```python
from build123d import *

# Parameters (mm, degrees)
BASPROSKE_W         = 15
BASPROSKE_H         = 20
TOOTHCUT_DEPTH      = 33.015621187
TEETHCUTS_COUNT     = 14
TEETHCUTS_ANGLE     = 334.285714286
BORSKE_R            = 2
BORE_DEPTH          = 50.0000508
SKETCH1_R           = 12.170076636
BOSS_EXTRUDE1_DEPTH = 20
SKETCH3_R           = 2
CUT_EXTRUDE1_DEPTH  = 45.828194428


with BuildPart() as part:
    # BasProSke → Base-Revolve (revolve)
    with BuildSketch(Plane(origin=(0, 0, 0), x_dir=(1, 0, 0), z_dir=(0, 1, 0)), mode=Mode.PRIVATE) as base_revolve_sk:
        with Locations((7.5, 10)):
            Rectangle(BASPROSKE_W, BASPROSKE_H)
    revolve(base_revolve_sk.sketch.rotate(Axis((-10, 0, 0), (1, 0, 0)), 180), axis=Axis((-10, 0, 0), (1, 0, 0)))

    # TooCutSke → ToothCut (cut, through all)
    with BuildSketch(Plane(origin=(0, 0, 0), x_dir=(0, 0, -1), z_dir=(1, 0, 0))):
        with BuildLine():
            ThreePointArc((1.339503949, 14.311450142), (0, 14.374), (-1.339503949, 14.311450142))
            ThreePointArc((-1.339503949, 14.311450142), (-2.055976555, 17.261705303), (-3.954182827, 19.631125371))
            ThreePointArc((-3.954182827, 19.631125371), (0, 20.0254), (3.954182827, 19.631125371))
            ThreePointArc((3.954182827, 19.631125371), (2.055976555, 17.261705303), (1.339503949, 14.311450142))
        make_face()
    toothcut = extrude(amount=TOOTHCUT_DEPTH, mode=Mode.SUBTRACT)

    # TeethCuts: ToothCut ×14 about axis
    teethcuts_axis = Axis((-10, 0, 0), (1, 0, 0))
    for i in range(1, TEETHCUTS_COUNT):
        add(toothcut.rotate(teethcuts_axis, i * TEETHCUTS_ANGLE / (TEETHCUTS_COUNT - 1)), mode=Mode.SUBTRACT)

    # BorSke → Bore (cut, symmetric)
    with BuildSketch(Plane(origin=(0, 0, 0), x_dir=(0, 0, -1), z_dir=(1, 0, 0))):
        with Locations(Location((0, 0, 0), (0, 0, 180))):
            Circle(BORSKE_R)
    extrude(amount=BORE_DEPTH, both=True, mode=Mode.SUBTRACT)

    # Sketch1 → Boss-Extrude1 (add)
    with BuildSketch(Plane(origin=(15, 0, 0), x_dir=(0, 0, -1), z_dir=(1, 0, 0))):
        with Locations(Location((0, 0, 0), (0, 0, 180))):
            Circle(SKETCH1_R)
    extrude(amount=BOSS_EXTRUDE1_DEPTH)

    # Sketch3 → Cut-Extrude1 (cut, through all)
    with BuildSketch(Plane(origin=(35, 0, 0), x_dir=(0, 0, -1), z_dir=(1, 0, 0))):
        Circle(SKETCH3_R)
    extrude(amount=-CUT_EXTRUDE1_DEPTH, mode=Mode.SUBTRACT)


solid = part.part
```
Could you check a few things on this model? Use its own coordinates, in mm. A direction names the side the tool comes from. Round coordinates to 2 decimals unless told otherwise and drop trailing zeros. Loops run counter-clockwise (first coordinate to the right, second up) from the corner with the lowest first, then second, coordinate; pieces in that order, holes last. Notation, with made-up numbers: (46.25, -28) - (87.25, -28) arc R30 ccw to (87.25, -6) - close; hole circle Ø7 at (36.25, -25.75). An arc over 180 degrees is marked (long way). Answer in a Markdown table with one row per item. Add a question column.
(1) If we section it at B-B (z = 0): Please give me the cut outline in (x, y).
(2) If we section it at A-A (y = 0): Please give me the cut outline in (x, z), plus the area to 3 significant figures.
(3) I'm going to push flat-ended pins straight in: pin 1 (10 mm diameter, centred on y = -7, z = -9.5, fed in from -X); pin 2 (6 mm diameter, centred on x = 6.5, y = -14.5, fed in from +Z); pin 3 (10 mm diameter, centred on x = 23.5, z = -11, fed in from -Y); pin 4 (4 mm diameter, centred on x = 20.5, y = 12, fed in from +Z). Where does each tip first touch, or does it pass through?
(4) I need wall thicknesses on line 1 along Y through (x, z) = (13, -10.5); line 2 along Y through (x, z) = (13.5, 0); line 3 along Y through (x, z) = (23, 0). Which ranges of each line are inside material? Lowest first, please.
(5) If we mould it in two halves opening along Y, with no side actions, what happens to faces 1 (the face through (7.6, -19.5, -4.44)), 2 (the face through (15, 8.4, 9.2)), 3 (the face through (7.4, 8.95, -11.25))? For each: pulls with the +Y half, pulls with the -Y half, needs draft (parallel to the pull), parting line crosses it, or undercut.
(6) If we section it at C-C (z = -11): Please give me the cut outline in (x, y), plus the area to 3 significant figures.
(7) For faces 4 (the face through (7.4, -12.32, 12.19)), 5 (the face through (7.4, 12.32, -12.19)), 6 (the face through (7.395, -14.624, -9.296)), 7 (the face through (7.395, 16.385, -5.637)), 8 (the face through (35, 3, 0)), which set-ups out of +Z, -Z, +X, -X, +Y, -Y let a thin tool reach every point of the face, with its end or its side?
(8) If we section it at D-D (x = 16.5): Please give me the cut outline in (y, z), plus the area to 3 significant figures.
Model answer:
| question | item | result |
|---|---|---|
| 1 | outline | (0, -14.37) - (15, -14.37) - (15, -12.17) - (35, -12.17) - (35, -2) - (0, -2) - close; (0, 2) - (35, 2) - (35, 12.17) - (15, 12.17) - (15, 14.37) - (0, 14.37) - close |
| 2 | outline | (0, -20) - (15, -20) - (15, -12.17) - (35, -12.17) - (35, -2) - (0, -2) - close; (0, 2) - (35, 2) - (35, 12.17) - (15, 12.17) - (15, 20) - (0, 20) - close |
| 2 | area | 947 mm² |
| 3 | pin 1 | stops at x = 0 |
| 3 | pin 2 | stops at z = 12.88 |
| 3 | pin 3 | stops at y = -10.59 |
| 3 | pin 4 | stops at z = 6.94 |
| 4 | line 1 | y = -15.4 to -10.09, -9.82 to 9.82, 10.09 to 15.4 |
| 4 | line 2 | y = -14.37 to -2, 2 to 14.37 |
| 4 | line 3 | y = -12.17 to -2, 2 to 12.17 |
| 5 | face 1 | pulls with the -Y half |
| 5 | face 2 | needs draft |
| 5 | face 3 | undercut |
| 6 | outline | (0, -15.63) - (15, -15.63) - (15, -10.58) - (0, -10.58) - close; (0, -9.25) - (15, -9.25) - (15, -5.21) - (35, -5.21) - (35, 5.21) - (15, 5.21) - (15, 9.25) - (0, 9.25) - close; (0, 10.58) - (15, 10.58) - (15, 15.63) - (0, 15.63) - close |
| 6 | area | 637 mm² |
| 7 | face 4 | +Z, +X, -X |
| 7 | face 5 | -Z, +X, -X |
| 7 | face 6 | +X, -X, -Y |
| 7 | face 7 | +X, -X |
| 7 | face 8 | +Z, -Z, +X, +Y, -Y |
| 8 | outline | circle Ø24.34 at (0, 0); hole circle Ø4 at (0, 0) |
| 8 | area | 453 mm² |
